Here's how the part is built. I have some questions about the finished solid (model axes, mm). A direction names the side the tool comes from. Coordinates: 2 decimals unless noted, no trailing zeros. Order: outer loops, then holes, each group sorted by start corner. A loop starts at its lowest first (then second) coordinate and runs counter-clockwise, first axis right, second up.
```python
from build123d import *

# Parameters (mm, degrees)
F0_R     = 6.35
F3_DEPTH = 30
F4_R     = 5


with BuildPart() as f2:
    # F1 (on Top) → F2 (revolve)
    with BuildSketch(Plane.XY):
        with BuildLine():
            Line((0, 19.451053), (0, -18.648947))
            ThreePointArc((0, -18.648947), (19.05, 0.401053), (0, 19.451053))
        make_face()
    revolve(axis=Axis((0, 0.401053, 0), (0, 1, 0)))

    # F0 (on Top) → F3 (join)
    with BuildSketch(Plane.XY):
        Circle(F0_R)
    extrude(amount=F3_DEPTH)

    # F4
    f4_edges = [f2.edges().sort_by_distance(p)[0] for p in [
        (19.05, 0.401053, 0),
        (-6.35, -1.7e-05, 17.956034),
        (-6.35, 0, 30),
    ]]
    fillet(f4_edges, radius=F4_R)


solid = f2.part
```
Q1. If we section it at B-B on y = 16.5: Write out the boundary of the cut face in (x, z), then the cut area to 3 significant figures.
Q2. For faces 1 (the flat face through (0, 0, 30)), 2 (the cylindrical face through (-1.38, -6.2, 22.96)), which set-ups out of +Z, -Z, +X, -X, +Y, -Y let a thin tool reach every point of the face, with its end or its side?
Q3. If we section it at A-A on z = 22: Write out the boundary of the cut face in (x, y).
Q4. I need wall thicknesses on L1, parallel to X at y = -5, z = 0; L2, parallel to Z at x = -4, y = 1; L3, parallel to Z at x = 0, y = -16.5. Which ranges of each line are inside material? Lowest first, please.
Q5. Will these pins go through, and if not, where does the flat tip stop? pin 1 (5 mm diameter, centred on x = -1, y = -13, fed in from +Z); pin 2 (3 mm diameter, centred on y = -9, z = 7, fed in from +X); pin 3 (1.5 mm diameter, centred on y = -9.5, z = 8, fed in from +X).
Reply:
1. outline: circle Ø20.37 at (0, 0)
1. area: 326 mm2
2. face 1: +Z, +X, -X, +Y, -Y
2. face 2: +Z
3. outline: circle Ø12.7 at (0, 0)
4. L1: x = -18.27 to 18.27
4. L2: z = -18.62 to 29.16
4. L3: z = -8.79 to 8.79
5. pin 1: stops at z = 15.6
5. pin 2: stops at x = 16.08
5. pin 3: stops at x = 14.81
